Could you check a few things on this model? Use its own coordinates, in mm. A direction names the side the tool comes from. Round coordinates to 2 decimals unless told otherwise and drop trailing zeros. Write each loop counter-clockwise with the first axis right and the second up, starting at its lowest first coordinate (ties: lowest second). Pieces come first, ordered by that corner, then holes. Notation, with made-up numbers: (68.25, -17.75) -> (103.25, -17.75) arc R16 cw to (103.25, -6.75) -> close; hole circle Ø7 at (48, -13.5). An arc over 180 degrees is marked (long way). Answer as CSV lines item,"result". Start each with the question number.
Q1. Imagine slicing it at A-A on x = -12. Please give me the cut outline in (y, z), and give its area (3 significant figures).
Q2. Will these pins go through, and if not, where does the flat tip stop? pin 1 Ø5 at (x, y) = (-12, 3.5) entering from +Z; pin 2 Ø2 at (y, z) = (90, 0.5) entering from -X.
Q3. For faces 4 (the flat face through (0, 109, 15)), 5 (the cylindrical face through (-7.493, 49.3, 0.33)), which set-ups out of +Z, -Z, +X, -X, +Y, -Y let a thin tool reach every point of the face, with its end or its side?
Q4. Imagine slicing it at D-D on y = 94. Please give me the cut outline in (x, z).
Q5. If I drill on line 1 (Y direction, x = 8.5, z = -5.25); line 2 (X direction, y = 109, z = 11); line 3 (Z direction, x = 2, y = 39), over which ranges is the centre line in solid material (lowest first)? Write a range as [from, to].
Q6. Imagine slicing it at C-C on x = 0. Please give me the cut outline in (y, z), and give its area (3 significant figures).
Q7. Imagine slicing it at B-B on z = -8.75. Please give me the cut outline in (x, y).
Q8. If we mould it in two halves opening along Y, with no side actions, what happens to faces 1 (the flat face through (8, 100, 0)), 2 (the flat face through (0, 109, -15)), 3 (the flat face through (0, 118, 0))? For each: pulls with the +Y half, pulls with the -Y half, needs draft (parallel to the pull), parting line crosses it, or undercut.
from build123d import *

# Parameters (mm, degrees)
F0_W     = 66
F0_H     = 30
F0_R     = 7.5
F1_DEPTH = 18
F3_R     = 1
F4_DEPTH = 70
F5_DEPTH = 100
F6_W     = 66
F6_H     = 30
F6_R     = 7.5
F7_DEPTH = 18
F8_R     = 1
F9_DEPTH = 70


# Not quite as in the source:
# - a feature names something its author has since deleted; it is built from what else it names


with BuildPart() as f1:
    # F0 (on Front) → F1 (new body)
    with BuildSketch(Plane.XZ):
        Rectangle(F0_W, F0_H)
        Circle(F0_R, mode=Mode.SUBTRACT)
        Circle(F0_R)
    extrude(amount=F1_DEPTH)

    # F3 (on offset) → F4 (join)
    with BuildSketch(Plane.YZ.offset(35)):
        with Locations((-9.0000117198, 0)):
            Circle(F3_R)
    extrude(amount=-F4_DEPTH)

    # F0 (on Front) → F5 (join)
    with BuildSketch(Plane.XZ):
        Circle(F0_R)
    extrude(amount=-F5_DEPTH)

    # F6 (on face) → F7 (join)
    with BuildSketch(Plane(origin=(0, 100, 0), x_dir=(-1, 0, 0), z_dir=(0, 1, 0))):
        Rectangle(F6_W, F6_H)
        Circle(F6_R, mode=Mode.SUBTRACT)
        Circle(F6_R)
    extrude(amount=F7_DEPTH)

    # F8 (on offset) → F9 (join)
    with BuildSketch(Plane.YZ.offset(35)):
        with Locations((109, 0)):
            Circle(F8_R)
    extrude(amount=-F9_DEPTH)


solid = f1.part
Checks:
1,outline,"(-18, -15) -> (0, -15) -> (0, 15) -> (-18, 15) -> close; (100, -15) -> (118, -15) -> (118, 15) -> (100, 15) -> close"
1,area,"1,080 mm^2"
2,pin 1,"through"
2,pin 2,"x = -7.5"
3,face 4,"+Z, +X, -X, +Y, -Y"
3,face 5,"none"
4,outline,"circle Ø15 at (0, 0)"
5,line 1,"[-18, 0], [100, 118]"
5,line 2,"[-33, 33]"
5,line 3,"[-7.23, 7.23]"
6,outline,"(-18, -15) -> (0, -15) -> (0, -7.5) -> (100, -7.5) -> (100, -15) -> (118, -15) -> (118, 15) -> (100, 15) -> (100, 7.5) -> (0, 7.5) -> (0, 15) -> (-18, 15) -> close"
6,area,"2,580 mm^2"
7,outline,"(-33, -18) -> (33, -18) -> (33, 0) -> (-33, 0) -> close; (-33, 100) -> (33, 100) -> (33, 118) -> (-33, 118) -> close"
8,face 1,"undercut"
8,face 2,"needs draft"
8,face 3,"pulls with the +Y half"
